from build123d import *

# Parameters (mm, degrees)
SCHIZZO1_W                   = 40
SCHIZZO1_H                   = 85
ESTRUSIONE_ESTRUSIONE1_DEPTH = 1
SCHIZZO2_R                   = 1.625
TAGLIO_ESTRUSIONE1_DEPTH     = 2
RIPETIZIONE_A_L1_COUNT       = 4
RIPETIZIONE_A_L1_PITCH       = 25


with BuildPart() as part:
    # Schizzo1 → Estrusione-Estrusione1 (new body, symmetric)
    with BuildSketch(Plane.XY):
        Rectangle(SCHIZZO1_W, SCHIZZO1_H)
    extrude(amount=ESTRUSIONE_ESTRUSIONE1_DEPTH, both=True)

    # Schizzo2 → Taglio-Estrusione1 (cut)
    with BuildSketch(Plane(origin=(0, 0, -1), x_dir=(-1, 0, 0), z_dir=(0, 0, -1))):
        with Locations((0, 37.5)):
            Circle(SCHIZZO2_R)
    taglio_estrusione1 = extrude(amount=-TAGLIO_ESTRUSIONE1_DEPTH, mode=Mode.SUBTRACT)

    # Ripetizione a L1: Taglio-Estrusione1 ×4
    with Locations(*[(0, -i * RIPETIZIONE_A_L1_PITCH, 0) for i in range(1, RIPETIZIONE_A_L1_COUNT)]):
        add(taglio_estrusione1, mode=Mode.SUBTRACT)


solid = part.part
Could you check a few things on this model? Use its own coordinates, in mm. Give positions to 0.01 mm unless a question says otherwise; leave off trailing zeros. Order: outer loops, then holes, each group sorted by start corner. A loop starts at its lowest first (then second) coordinate and runs counter-clockwise, first axis right, second up. Notation, with made-up numbers: (42, 1.25) -> (61, 1.25) arc R13 ccw to (61, 14.25) -> close; hole circle Ø3 at (52, 48). An arc over 180 degrees is marked (long way). Answer in a Markdown table with one row per item. Add a question column.
Item 1: Imagine slicing it at B-B (x = 0). List the corners of the cut face in (y, z) for me (3 decimals).
Item 2: Imagine slicing it at A-A (y = -12.5). List the corners of the cut face in (x, z) for me (3 decimals), and give its area (3 significant figures).
Item 3: I'm going to push a flat-ended pin straight in: P1, Ø3, axis at x = 0, y = 12.5, coming from the -Z side. Where does the tip first touch, or does it pass through?
Item 4: We'd pull the mould along X, two halves only. Please class faces 1 (the flat face through (0, 1, -1)), 2 (the cylindrical face through (1.198, 13.598, -0.014)), 3 (the flat face through (-20, -1, 0)): pulls with the +X half, pulls with the -X half, needs draft (parallel to the pull), parting line crosses it, or undercut.
Item 5: Please list where these lines run through material, in increasing order: probe 1 along Y at (x, z) = (0, 0.05) (3 decimals); probe 2 along X at (y, z) = (-13.5, -0.1).
Result:
| question | item | result |
|---|---|---|
| 1 | outline | (-42.5, -1) -> (-39.125, -1) -> (-39.125, 1) -> (-42.5, 1) -> close; (-35.875, -1) -> (-14.125, -1) -> (-14.125, 1) -> (-35.875, 1) -> close; (-10.875, -1) -> (10.875, -1) -> (10.875, 1) -> (-10.875, 1) -> close; (14.125, -1) -> (35.875, -1) -> (35.875, 1) -> (14.125, 1) -> close; (39.125, -1) -> (42.5, -1) -> (42.5, 1) -> (39.125, 1) -> close |
| 2 | outline | (-20, -1) -> (-1.625, -1) -> (-1.625, 1) -> (-20, 1) -> close; (1.625, -1) -> (20, -1) -> (20, 1) -> (1.625, 1) -> close |
| 2 | area | 73.5 mm2 |
| 3 | P1 | through |
| 4 | face 1 | needs draft |
| 4 | face 2 | undercut |
| 4 | face 3 | pulls with the -X half |
| 5 | probe 1 | -42.5 to -39.125, -35.875 to -14.125, -10.875 to 10.875, 14.125 to 35.875, 39.125 to 42.5 |
| 5 | probe 2 | -20 to -1.28, 1.28 to 20 |
